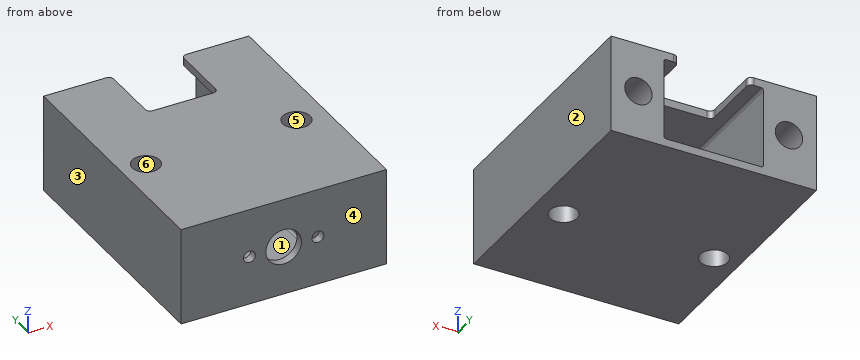
from build123d import *

# Parameters (mm, degrees)
F0_R     = 1.778
F0_W     = 9.144
F0_H     = 1.016
F0_R_2   = 0.76835
F0_R_3   = 2.3114
F1_DEPTH = 32.512
F2_DEPTH = 31.4325
F3_DEPTH = 8.6995
F4_DEPTH = 8.89
F5_R     = 1.778
F6_DEPTH = 12.701
F7_R     = 0.635


with BuildPart() as f1:
    # F0 (on Front) → F1 (new body)
    with BuildSketch(Plane.XZ):
        with BuildLine():
            Line((-13.335, -6.35), (13.335, -6.35))
            Line((13.335, -6.35), (13.335, 6.35))
            Line((13.335, 6.35), (4.572, 6.35))
            Line((4.572, 6.35), (4.572, 5.334))
            Line((4.572, 5.334), (6.159687, 5.334))
            ThreePointArc((6.159687, 5.334), (6.384061, 5.241061), (6.477, 5.016687))
            Line((6.477, 5.016687), (6.477, -5.016687))
            ThreePointArc((6.477, -5.016687), (6.384061, -5.241061), (6.159687, -5.334))
            Line((6.159687, -5.334), (-6.159687, -5.334))
            ThreePointArc((-6.159687, -5.334), (-6.384061, -5.241061), (-6.477, -5.016687))
            Line((-6.477, -5.016687), (-6.477, 5.016687))
            ThreePointArc((-6.477, 5.016687), (-6.384061, 5.241061), (-6.159687, 5.334))
            Line((-6.159687, 5.334), (-4.572, 5.334))
            Line((-4.572, 5.334), (-4.572, 6.35))
            Line((-4.572, 6.35), (-13.335, 6.35))
            Line((-13.335, 6.35), (-13.335, -6.35))
        make_face()
        with Locations((-9.779, 0)):
            Circle(F0_R, mode=Mode.SUBTRACT)
        with Locations((9.779, 0)):
            Circle(F0_R, mode=Mode.SUBTRACT)
        with Locations((0, 5.842)):
            Rectangle(F0_W, F0_H)
        with BuildLine():
            Line((6.159687, 5.334), (4.572, 5.334))
            Line((4.572, 5.334), (-4.572, 5.334))
            Line((-4.572, 5.334), (-6.159687, 5.334))
            ThreePointArc((-6.159687, 5.334), (-6.384061, 5.241061), (-6.477, 5.016687))
            Line((-6.477, 5.016687), (-6.477, -5.016687))
            ThreePointArc((-6.477, -5.016687), (-6.384061, -5.241061), (-6.159687, -5.334))
            Line((-6.159687, -5.334), (6.159687, -5.334))
            ThreePointArc((6.159687, -5.334), (6.384061, -5.241061), (6.477, -5.016687))
            Line((6.477, -5.016687), (6.477, 5.016687))
            ThreePointArc((6.477, 5.016687), (6.384061, 5.241061), (6.159687, 5.334))
        make_face()
        with Locations((-4.445, 0)):
            Circle(F0_R_2, mode=Mode.SUBTRACT)
        Circle(F0_R_3, mode=Mode.SUBTRACT)
        with Locations((4.445, 0)):
            Circle(F0_R_2, mode=Mode.SUBTRACT)
        with Locations((-9.779, 0)):
            Circle(F0_R)
        with Locations((9.779, 0)):
            Circle(F0_R)
    extrude(amount=F1_DEPTH)

    # F0 (on Front) → F2 (cut)
    with BuildSketch(Plane.XZ):
        with BuildLine():
            Line((6.159687, 5.334), (4.572, 5.334))
            Line((4.572, 5.334), (-4.572, 5.334))
            Line((-4.572, 5.334), (-6.159687, 5.334))
            ThreePointArc((-6.159687, 5.334), (-6.384061, 5.241061), (-6.477, 5.016687))
            Line((-6.477, 5.016687), (-6.477, -5.016687))
            ThreePointArc((-6.477, -5.016687), (-6.384061, -5.241061), (-6.159687, -5.334))
            Line((-6.159687, -5.334), (6.159687, -5.334))
            ThreePointArc((6.159687, -5.334), (6.384061, -5.241061), (6.477, -5.016687))
            Line((6.477, -5.016687), (6.477, 5.016687))
            ThreePointArc((6.477, 5.016687), (6.384061, 5.241061), (6.159687, 5.334))
        make_face()
        with Locations((-4.445, 0)):
            Circle(F0_R_2, mode=Mode.SUBTRACT)
        Circle(F0_R_3, mode=Mode.SUBTRACT)
        with Locations((4.445, 0)):
            Circle(F0_R_2, mode=Mode.SUBTRACT)
    extrude(amount=F2_DEPTH, mode=Mode.SUBTRACT)

    # F0 (on Front) → F3 (cut)
    with BuildSketch(Plane.XZ):
        with Locations((0, 5.842)):
            Rectangle(F0_W, F0_H)
    extrude(amount=F3_DEPTH, mode=Mode.SUBTRACT)

    # F0 (on Front) → F4 (cut)
    with BuildSketch(Plane.XZ):
        with Locations((9.779, 0)):
            Circle(F0_R)
        with Locations((-9.779, 0)):
            Circle(F0_R)
    extrude(amount=F4_DEPTH, mode=Mode.SUBTRACT)

    # F5 (on face) → F6 (cut, through all)
    with BuildSketch(Plane.XY.offset(6.35)):
        with Locations((-10.089038, -18.288)):
            Circle(F5_R)
        with Locations((9.468962, -18.288)):
            Circle(F5_R)
    extrude(amount=-F6_DEPTH, mode=Mode.SUBTRACT)

    # F7
    f7_edges = [f1.edges().sort_by_distance(p)[0] for p in [
        (-4.572, -8.6995, 5.842),
        (4.572, -8.6995, 5.842),
        (4.572, 0, 5.842),
        (-4.572, 0, 5.842),
    ]]
    fillet(f7_edges, radius=F7_R)


solid = f1.part
Check sheet for the modelled part. Datum: model origin and axes. Units: mm. Face numbers are marked on the shaded views. A direction names the side the tool comes from. Round coordinates to 2 decimals unless told otherwise and drop trailing zeros. Write each loop counter-clockwise with the first axis right and the second up, starting at its lowest first coordinate (ties: lowest second). Pieces come first, ordered by that corner, then holes. Notation, with made-up numbers: (20.5, -36) - (73.5, -36) arc R29 ccw to (73.5, -13) - close; hole circle Ø5 at (82, 40.25). An arc over 180 degrees is marked (long way). Return JSON: item names as keys, results as strings.
Q1. Cross-section at A-A (x = 0). Record the boundary of the cut face in (y, z), then the cut area to 3 significant figures.
Returned:
{"outline": "(-32.51, -6.35) - (0, -6.35) - (0, -5.33) - (-31.43, -5.33) - (-31.43, -2.31) - (-32.51, -2.31) - close; (-32.51, 2.31) - (-31.43, 2.31) - (-31.43, 5.33) - (-8.7, 5.33) - (-8.7, 6.35) - (-32.51, 6.35) - close", "area": "63.8 mm²"}
Q2. Access from +Z, -Z, +X, -X, +Y, -Y to the whole of each face (thin tool, end or side, straight path). Record for the marked faces 1 and 2.
Returned:
{"face 1": "+Y", "face 2": "+Z, -Z, +X, +Y, -Y"}
Q3. Cross-section at D-D (z = -3.75). Record the boundary of the cut face in (x, y) (1 decimal).
Returned:
{"outline": "(-13.3, -32.5) - (13.3, -32.5) - (13.3, 0) - (6.5, 0) - (6.5, -31.4) - (-6.5, -31.4) - (-6.5, 0) - (-13.3, 0) - close; hole circle Ø3.6 at (-10.1, -18.3); hole circle Ø3.6 at (9.5, -18.3)"}
Q4. Scan lines: L1, parallel to X at y = -14, z = 5 (3 decimals); L2, parallel to Z at x = -5.5, y = -6; L3, parallel to X at y = -8.5, z = -1 (3 decimals). Record each from-to range of solid material in increasing order. Write a range as from..to.
Returned:
{"L1": "x = -13.335..-6.477, 6.477..13.335", "L2": "z = -6.35..-5.33, 5.33..6.35", "L3": "x = -13.335..-11.249, -8.309..-6.477, 6.477..8.309, 11.249..13.335"}
Q5. Draft check along Y on the marked faces 3, 4, 5 and 6. Enter one of: released by +Y, released by -Y, zero draft, split by the parting line, or undercut.
Returned:
{"face 3": "zero draft", "face 4": "released by -Y", "face 5": "undercut", "face 6": "undercut"}
Q6. Cross-section at C-C (z = 0). Give the number of separate pieces and of enclosed holes in the cut face, then the cut area to 3 significant figures.
Returned:
{"separate pieces": "4", "enclosed holes": "2", "area": "369 mm²"}
Q7. Depth check by flat-ended pin: P1, Ø5.5, axis at x = 3, z = 2, coming from the +Y side; P2, Ø0.8, axis at x = 1.5, z = 6, coming from the +Y side; P3, Ø3, axis at x = 9.47, y = -18.29, coming from the -Z side. Enter the tip coordinate at first touch or a pass-through.
Returned:
{"P1": "stops at y = -31.43", "P2": "stops at y = -8.7", "P3": "passes through"}
Q8. Cross-section at B-B (y = -19.5). Record the boundary of the cut face in (x, z) (3 decimals), then the cut area to 3 significant figures.
Returned:
{"outline": "(-13.335, -6.35) - (-11.39, -6.35) - (-11.39, 6.35) - (-13.335, 6.35) - close; (-8.788, -6.35) - (8.168, -6.35) - (8.168, 6.35) - (-8.788, 6.35) - close; (10.77, -6.35) - (13.335, -6.35) - (13.335, 6.35) - (10.77, 6.35) - close; hole (-6.477, -5.017) arc R0.317 ccw to (-6.16, -5.334) - (6.16, -5.334) arc R0.317 ccw to (6.477, -5.017) - (6.477, 5.017) arc R0.317 ccw to (6.16, 5.334) - (-6.16, 5.334) arc R0.317 ccw to (-6.477, 5.017) - close", "area": "135 mm²"}
